The model under review builds one solid part; all positions refer to its coordinate system, in mm. A direction names the side the tool comes from. Round coordinates to 2 decimals unless told otherwise and drop trailing zeros. Order: outer loops, then holes, each group sorted by start corner. A loop starts at its lowest first (then second) coordinate and runs counter-clockwise, first axis right, second up. Notation, with made-up numbers: (5, 81.25) -> (13, 81.25) arc R20 cw to (13, 103.25) -> close; hole circle Ø1 at (86.25, 87). An arc over 180 degrees is marked (long way). Return JSON: item names as keys, results as strings. Group by question number.
from build123d import *

# Parameters (mm, degrees)
F0_W     = 20.5
F0_H     = 40.7
F1_DEPTH = 35
F2_R     = 1.651
F3_DEPTH = 6.35
F4_W     = 20.5
F4_H     = 5
F5_DEPTH = 6.5
F6_W     = 20.5
F6_H     = 5
F7_DEPTH = 6.5
F8_SIZE  = 1.397


with BuildPart() as f1:
    # F0 (on Top) → F1 (new body)
    with BuildSketch(Plane.XY):
        Rectangle(F0_W, F0_H)
    extrude(amount=F1_DEPTH)

    # F2 (on face) → F3 (join)
    with BuildSketch(Plane.XY.offset(35)):
        with Locations((0, -10.825)):
            Circle(F2_R)
    extrude(amount=F3_DEPTH)

    # F4 (on face) → F5 (join)
    with BuildSketch(Plane.XZ.offset(20.35)):
        with Locations((0, 27.5)):
            Rectangle(F4_W, F4_H)
    extrude(amount=F5_DEPTH)

    # F6 (on face) → F7 (join)
    with BuildSketch(Plane(origin=(0, 20.35, 0), x_dir=(-1, 0, 0), z_dir=(0, 1, 0))):
        with Locations((0, 27.5)):
            Rectangle(F6_W, F6_H)
    extrude(amount=F7_DEPTH)

    # F8
    f8_edges = [f1.edges().sort_by_distance(p)[0] for p in [
        (0, -20.35, 0),
        (10.25, 0, 0),
        (-10.25, 0, 0),
        (0, 20.35, 0),
    ]]
    chamfer(f8_edges, length=F8_SIZE)


solid = f1.part
Item 1: Consider section A-A on x = -7.75. State the section outline as (y, z) points, plus the area to 3 significant figures.
Item 2: Consider section B-B on y = 10.5. State the section outline as (x, z) points.
Item 3: Wall thickness on line 1 along Y through (x, z) = (6.25, 16); line 2 along Z through (x, y) = (-8.75, -5); line 3 along Z through (x, y) = (2.5, -20): over which ranges is each line inside the solid? List them lowest first.
Item 4: Insertion check: pin 1 Ø5.5 at (x, z) = (3.5, 31.5) entering from -Y; pin 2 Ø1 at (x, z) = (3.5, 13) entering from +Y; pin 3 Ø5 at (x, y) = (2.5, -24.5) entering from +Z; pin 4 Ø12 at (x, z) = (-5.5, 6.5) entering from -Y. Each pin has a flat end and moves straight along its axis. Give the tip position at first contact, or say it passes through.
Item 5: Consider section D-D on x = 0. State the section outline as (y, z) points, plus the area to 3 significant figures.
Item 6: For faces 1 (the face through (0, -24, 30)), 2 (the face through (0, 20.35, 32)), 3 (the face through (0, -24, 25)), list the 3-axis set-ups (+Z, -Z, +X, -X, +Y, -Y) from which the entire face can be reached by the end or side of a thin tool; tool diameter is ignored.
Item 7: Consider section C-C on z = 20. State the section outline as (x, y) points.
Values:
{
 "1": {"outline": "(-26.85, 25) -> (-20.35, 25) -> (-20.35, 1.4) -> (-18.95, 0) -> (18.95, 0) -> (20.35, 1.4) -> (20.35, 25) -> (26.85, 25) -> (26.85, 30) -> (20.35, 30) -> (20.35, 35) -> (-20.35, 35) -> (-20.35, 30) -> (-26.85, 30) -> close", "area": "1,490 mm^2"},
 "2": {"outline": "(-10.25, 1.4) -> (-8.85, 0) -> (8.85, 0) -> (10.25, 1.4) -> (10.25, 35) -> (-10.25, 35) -> close"},
 "3": {"line 1": "-20.35 to 20.35", "line 2": "0 to 35", "line 3": "1.05 to 35"},
 "4": {"pin 1": "y = -26.85", "pin 2": "y = 20.35", "pin 3": "z = 30", "pin 4": "y = -20.35"},
 "5": {"outline": "(-26.85, 25) -> (-20.35, 25) -> (-20.35, 1.4) -> (-18.95, 0) -> (18.95, 0) -> (20.35, 1.4) -> (20.35, 25) -> (26.85, 25) -> (26.85, 30) -> (20.35, 30) -> (20.35, 35) -> (-9.17, 35) -> (-9.17, 41.35) -> (-12.48, 41.35) -> (-12.48, 35) -> (-20.35, 35) -> (-20.35, 30) -> (-26.85, 30) -> close", "area": "1,510 mm^2"},
 "6": {"face 1": "+Z, +X, -X, -Y", "face 2": "+Z, +X, -X, +Y", "face 3": "-Z, +X, -X, -Y"},
 "7": {"outline": "(-10.25, -20.35) -> (10.25, -20.35) -> (10.25, 20.35) -> (-10.25, 20.35) -> close"}
}
